Read the model definition and answer for the solid it produces. Units are mm, in the model's axes. Face numbers are marked on the shaded views. A direction names the side the tool comes from. Coordinates: 2 decimals unless noted, no trailing zeros. Loops run counter-clockwise (first coordinate to the right, second up) from the corner with the lowest first, then second, coordinate; pieces in that order, holes last.
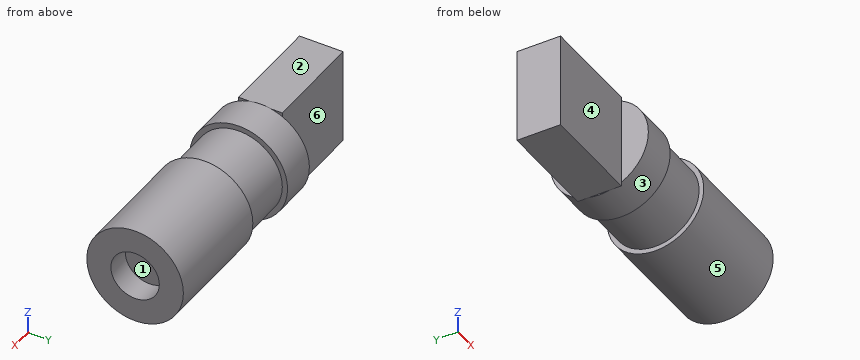
Autodesk Inventor part; units mm, degrees
ref_plane "YZ Plane" through (0, 0, 0) normal (1, 0, 0) x (0, 1, 0)
ref_plane "XZ Plane" through (0, 0, 0) normal (0, 1, 0) x (-1, 0, 0)
ref_plane "XY Plane" through (0, 0, 0) normal (0, 0, 1) x (1, 0, 0)
sketch "Sketch1" plane through (0, 0, 0) normal (0, 0, 1) x (1, 0, 0)
  line L0 (0, 0) -> (11.5, 0)
  line L1 (13, 1.5) -> (13, 2.99)
  line L2 (13, 2.99) -> (5.8, 2.99)
  line L3 (5.8, 2.99) -> (5.8, 2.7)
  line L4 (5.8, 2.7) -> (2.26, 2.7)
  line L5 (2.26, 2.7) -> (2.26, 3.025)
  line L6 (2.26, 3.025) -> (0, 3.025)
  line L7 (0, 3.025) -> (0, 0)
  line L8 (13, 1.5) -> (11.5, 1.5)
  line L9 (11.5, 1.5) -> (11.5, 0)
  dimension "d0" = 7.2
  dimension "d1" = 5.98
  dimension "d2" = 2.26
  dimension "d3" = 6.05
  dimension "d4" = 3
  dimension "d5" = 1.5
  dimension "d6" = 13
  dimension "d7" = 5.4
revolve "Revolution1" add sketch "Sketch1" angle 360 about axis through (0, 0, 0) along (1, 0, 0)
sketch "Sketch2" plane through (0, 0, 0) normal (-1, 0, 0) x (0, 0, 1)
  line L0 (-2.95, -1.35) -> (2.95, -1.35)
  line L1 (2.95, -1.35) -> (2.95, 1.35)
  line L2 (2.95, 1.35) -> (-2.95, 1.35)
  line L3 (-2.95, 1.35) -> (-2.95, -1.35)
  line L4 (-2.95, -1.35) -> (2.95, 1.35) construction
  line L5 (2.95, -1.35) -> (-2.95, 1.35) construction
  point P0 (0, 0)
  dimension "d9" = 5.9
  dimension "d10" = 2.7
extrude "Extrusion1" add sketch "Sketch2" along normal blind 6.3
properties part number "laser_taida_6mm" material "Brass, Soft Yellow"
Q1. Flat-ended cylindrical pins translate along their axes: pin 1 Ø1.4 at (x, y) = (-3.5, 0) entering from +Z; pin 2 Ø3 at (x, z) = (5, 2.5) entering from -Y; pin 3 Ø1.8 at (x, z) = (-3, 1) entering from +Y. Find the tip coordinate at first contact, or state that the pin passes through.
Findings below:
pin 1: stops at z = 2.95
pin 2: stops at y = -2.72
pin 3: stops at y = 1.35
Q2. A cutting plane is placed at A-A (y = 0). Give the vertices of the cut face in (x, z) (3 decimals), then the cut area to 3 significant figures.
Findings below:
outline: (-6.3, -2.95) - (0, -2.95) - (0, -3.025) - (2.26, -3.025) - (2.26, -2.7) - (5.8, -2.7) - (5.8, -2.99) - (13, -2.99) - (13, -1.5) - (11.5, -1.5) - (11.5, 1.5) - (13, 1.5) - (13, 2.99) - (5.8, 2.99) - (5.8, 2.7) - (2.26, 2.7) - (2.26, 3.025) - (0, 3.025) - (0, 2.95) - (-6.3, 2.95) - close
area: 109 mm2
Q3. A cutting plane is placed at C-C (x = -3). Give the vertices of the cut face in (y, z), then the cut area to 3 significant figures.
Findings below:
outline: (-1.35, -2.95) - (1.35, -2.95) - (1.35, 2.95) - (-1.35, 2.95) - close
area: 15.9 mm2
Q4. Straight lines are drawn through the part: probe 1 along Z at (x, y) = (11.8, 0); probe 2 along X at (y, z) = (-1.5, -2.5); probe 3 along X at (y, z) = (-2, -1.5). For each, find the intervals that lie inside material, in ascending order.
Findings below:
probe 1: z = -2.99 to -1.5, 1.5 to 2.99
probe 2: x = 0 to 2.26, 5.8 to 13
probe 3: x = 0 to 13
Q5. A cutting plane is placed at B-B (z = 0). Give the vertices of the cut face in (x, y) (3 decimals).
Findings below:
outline: (-6.3, -1.35) - (0, -1.35) - (0, -3.025) - (2.26, -3.025) - (2.26, -2.7) - (5.8, -2.7) - (5.8, -2.99) - (13, -2.99) - (13, -1.5) - (11.5, -1.5) - (11.5, 1.5) - (13, 1.5) - (13, 2.99) - (5.8, 2.99) - (5.8, 2.7) - (2.26, 2.7) - (2.26, 3.025) - (0, 3.025) - (0, 1.35) - (-6.3, 1.35) - close
Q6. Determine the mould class of the marked faces 1, 2 and 3 for opening direction Y: +Y half, -Y half, draft (parallel to the pull), parting line (faces both ways), or undercut.
Findings below:
face 1: undercut
face 2: draft
face 3: parting line
Q7. A cutting plane is placed at D-D (z = 2). Give the vertices of the cut face in (x, y).
Findings below:
outline: (-6.3, -1.35) - (0, -1.35) - (0, -2.27) - (2.26, -2.27) - (2.26, -1.81) - (5.8, -1.81) - (5.8, -2.22) - (13, -2.22) - (13, 2.22) - (5.8, 2.22) - (5.8, 1.81) - (2.26, 1.81) - (2.26, 2.27) - (0, 2.27) - (0, 1.35) - (-6.3, 1.35) - close
Q8. Which of the six approach directions +Z, -Z, +X, -X, +Y, -Y give full straight-line access (tool end or side, diameter ignored) to the marked faces 4, 5 and 6?
Findings below:
face 4: +Z, -Z, -X, -Y
face 5: +X
face 6: +Z, -Z, -X, +Y
